Design review of the part built by this model. Coordinates are the model's own, in mm. Give positions to 0.01 mm unless a question says otherwise; leave off trailing zeros. Write each loop counter-clockwise with the first axis right and the second up, starting at its lowest first coordinate (ties: lowest second). Pieces come first, ordered by that corner, then holes. Notation, with made-up numbers: (21.25, -40) -> (33.25, -40) arc R24 ccw to (33.25, -22) -> close; hole circle Ø3 at (-15, 37.25). An arc over 180 degrees is marked (long way). Put each result on its own line as item: value. Start each with the question number.
from build123d import *

# Parameters (mm, degrees)
F0_W           = 158.75
F0_H           = 76.2
F1_DEPTH       = 9
F3_D           = 9
F3_CSINK_D     = 17.92
F3_CSINK_ANGLE = 90
F5_D           = 3.3


with BuildPart() as f1:
    # F0 (on Top) → F1 (new body, symmetric)
    with BuildSketch(Plane.XY):
        Rectangle(F0_W, F0_H)
    extrude(amount=F1_DEPTH, both=True)

    # F3 (through all)
    with Locations(Plane.XY.offset(9)):
        with Locations((-60, 0), (60, 0)):
            CounterSinkHole(F3_D / 2, F3_CSINK_D / 2, counter_sink_angle=F3_CSINK_ANGLE)

    # F5 (through all)
    with Locations(Plane.XY.offset(9)):
        with Locations((-54.375, 20.1), (17.625, 28.1), (17.625, -26.9)):
            Hole(F5_D / 2)


solid = f1.part
Q1. Take a section at C-C on x = -60. Give the boundary of the cut face in (y, z), then the cut area to 3 significant figures.
Q2. Take a section at B-B on z = 6.25. Give the boundary of the cut face in (x, y) (3 decimals).
Q3. Take a section at A-A on y = -26.9. Give the boundary of the cut face in (x, z) (3 decimals), then the cut area to 3 significant figures.
Q4. For pin 1 (11.5 mm diameter, centred on x = -60, y = 0, fed in from +Z), flat-tipped, find the tip position at first contact; note if it passes through.
Q5. Mouldability with a two-part tool opening along Y and no side actions: class faces 1 (the face through (-1, 1, 9)), 2 (the face through (64.712, 0.207, 4.757)), 3 (the face through (-1, -38.1, 0)), 4 (the face through (-55.288, 0.207, 4.757)) as +Y half, -Y half, draft (parallel to the pull), parting line (faces both ways), or undercut.
Q6. To check wall thickness, follow probe 1 along X at (y, z) = (0, -4.25) (3 decimals); probe 2 along Y at (x, z) = (58.5, -6.5); probe 3 along Y at (x, z) = (-56.5, 4.75). State the ranges of each line that lie inside material, in increasing order. Write a range as from..to.
Result:
1. outline: (-38.1, -9) -> (-4.5, -9) -> (-4.5, 4.54) -> (-8.96, 9) -> (-38.1, 9) -> close; (4.5, -9) -> (38.1, -9) -> (38.1, 9) -> (8.96, 9) -> (4.5, 4.54) -> close
1. area: 1,190 mm^2
2. outline: (-79.375, -38.1) -> (79.375, -38.1) -> (79.375, 38.1) -> (-79.375, 38.1) -> close; hole circle Ø12.42 at (-60, 0); hole circle Ø3.3 at (-54.375, 20.1); hole circle Ø3.3 at (17.625, -26.9); hole circle Ø3.3 at (17.625, 28.1); hole circle Ø12.42 at (60, 0)
3. outline: (-79.375, -9) -> (15.975, -9) -> (15.975, 9) -> (-79.375, 9) -> close; (19.275, -9) -> (79.375, -9) -> (79.375, 9) -> (19.275, 9) -> close
3. area: 2,800 mm^2
4. pin 1: stops at z = 5.79
5. face 1: draft
5. face 2: undercut
5. face 3: -Y half
5. face 4: undercut
6. probe 1: x = -79.375..-64.5, -55.5..55.5, 64.5..79.375
6. probe 2: y = -38.1..-4.24, 4.24..38.1
6. probe 3: y = -38.1..-3.15, 3.15..38.1
